```python
from build123d import *

# Parameters (mm, degrees)
F1_DEPTH  = 50
F2_R      = 20
F3_DEPTH  = 25
F6_R      = 0.75
F7_DEPTH  = 25
F9_DEPTH  = 2
F10_R     = 0.75
F11_DEPTH = 5


# Not quite as in the source:
# - the program builds the solid bodies; features that only make, move or delete a surface that nothing else refers to are left out


with BuildPart() as f1:
    # F0 (on Top) → F1 (new body)
    with BuildSketch(Plane.XY):
        with BuildLine():
            Line((16.436829567, 25), (-13.563170433, 25))
            ThreePointArc((-13.563170433, 25), (-20.6342382449, 22.0710678119), (-23.563170433, 15))
            Line((-23.563170433, 15), (-23.563170433, -15))
            ThreePointArc((-23.563170433, -15), (-20.6342382449, -22.0710678119), (-13.563170433, -25))
            Line((-13.563170433, -25), (16.436829567, -25))
            ThreePointArc((16.436829567, -25), (23.5078973788, -22.0710678119), (26.436829567, -15))
            Line((26.436829567, -15), (26.436829567, 15))
            ThreePointArc((26.436829567, 15), (23.5078973788, 22.0710678119), (16.436829567, 25))
        make_face()
    extrude(amount=F1_DEPTH)

    # F2 (on face) → F3 (cut)
    with BuildSketch(Plane.XY.offset(50)):
        Circle(F2_R)
    extrude(amount=-F3_DEPTH, mode=Mode.SUBTRACT)

    # F4 (on Front) → F5 (revolve, cut)
    with BuildSketch(Plane.XZ):
        Polygon((20, 48), (20, 50), (0, 50), (0, 25), (23, 25), (23, 48), align=None)
    revolve(axis=Axis((0, 0, 37.5), (0, 0, 1)), mode=Mode.SUBTRACT)

    # F6 (on face) → F7 (cut)
    with BuildSketch(Plane.XY.offset(50)):
        with Locations((0, 21.75)):
            Circle(F6_R)
        with Locations((0, -21.75)):
            Circle(F6_R)
    extrude(amount=-F7_DEPTH, mode=Mode.SUBTRACT)

    # F8 (on face) → F9 (cut)
    with BuildSketch(Plane.XY.offset(25)):
        with BuildLine():
            ThreePointArc((7, 4), (6.7071067812, 4.7071067812), (6, 5))
            Line((6, 5), (-6, 5))
            ThreePointArc((-6, 5), (-6.7071067812, 4.7071067812), (-7, 4))
            Line((-7, 4), (-7, -4))
            ThreePointArc((-7, -4), (-6.7071067812, -4.7071067812), (-6, -5))
            Line((-6, -5), (6, -5))
            ThreePointArc((6, -5), (6.7071067812, -4.7071067812), (7, -4))
            Line((7, -4), (7, 4))
        make_face()
    extrude(amount=-F9_DEPTH, mode=Mode.SUBTRACT)

    # F10 (on face) → F11 (cut)
    with BuildSketch(Plane.XY.offset(23)):
        with Locations((-5.4101994716, 3.5321465987)):
            Circle(F10_R)
        with Locations((-5.4101994716, -3.5321465987)):
            Circle(F10_R)
        with Locations((5.4101994716, 3.5321465987)):
            Circle(F10_R)
        with Locations((5.4101994716, -3.5321465987)):
            Circle(F10_R)
    extrude(amount=-F11_DEPTH, mode=Mode.SUBTRACT)


solid = f1.part
```
Here's how the part is built. I have some questions about the finished solid (model axes, mm). A direction names the side the tool comes from. Give positions to 0.01 mm unless a question says otherwise; leave off trailing zeros. Loops run counter-clockwise (first coordinate to the right, second up) from the corner with the lowest first, then second, coordinate; pieces in that order, holes last. Notation, with made-up numbers: M 8,-37.5 L 43,-37.5 A25 cw 43,-8.5 Z; hole C 28,-18.75 d10. An arc over 180 degrees is marked long. Use one line per item in the form item = value. Start each with the question number.
Q1. If we section it at B-B (x = 0): Write out the boundary of the cut face in (y, z), then the cut area to 3 significant figures.
Q2. If we section it at A-A (z = 33): Write out the boundary of the cut face in (x, y), then the cut area to 3 significant figures.
Q3. Will these pins go through, and if not, where does the flat tip stop? pin 1 Ø12 at (x, y) = (-7, -10.5) entering from +Z; pin 2 Ø1.2 at (x, y) = (5.41, 3.53) entering from -Z; pin 3 Ø1.2 at (x, y) = (-5.41, -3.53) entering from +Z; pin 4 Ø2 at (x, z) = (-17.5, 34.5) entering from +Y.
Q4. Thinking about a two-plate mould opening in Y: for faces 1 (the cylindrical face through (5.31, -2.79, 20.54)), 2 (the flat face through (7, 0, 24)), 3 (the flat face through (-23.563, 0, 25)), 4 (the cylindrical face through (-20.556, 22.148, 24.65)), which applies, +Y half, -Y half, draft (parallel to the pull), parting line (faces both ways), or undercut?
Q5. If we section it at D-D (y = 0): Write out the boundary of the cut face in (x, z).
Q6. I need wall thicknesses on line 1 along Z through (x, y) = (9, -19); line 2 along Z through (x, y) = (11.5, 8.5); line 3 along X through (y, z) = (-17, 27.5). Which ranges of each line are inside material? Lowest first, please.
Q7. If we section it at C-C (z = 8): Write out the boundary of the cut face in (x, y).
Q8. Which directions (+Z, -Z, +X, -X, +Y, -Y) give clear straight access to the entire face, cutting with the end or side of a thin tool? Please do faces 5 (the flat face through (26.437, 0, 25)), 6 (the cylindrical face through (-2.994, 22.804, 36.661)), 7 (the cylindrical face through (0, 21, 49)).
Taken from the geometry:
q1.outline = M -25,0 L 25,0 L 25,50 L 22.5,50 L 22.5,48 L 23,48 L 23,25 L 5,25 L 5,23 L -5,23 L -5,25 L -23,25 L -23,48 L -22.5,48 L -22.5,50 L -25,50 Z; M -21,48 L -20,48 L -20,50 L -21,50 Z; M 20,48 L 21,48 L 21,50 L 20,50 Z
q1.area = 1,340 mm^2
q2.outline = M -23.56,-15 A10 ccw -13.56,-25 L 16.44,-25 A10 ccw 26.44,-15 L 26.44,15 A10 ccw 16.44,25 L -13.56,25 A10 ccw -23.56,15 Z; hole C 0,0 d46
q2.area = 752 mm^2
q3.pin_1 = 25
q3.pin_2 = 0
q3.pin_3 = 18
q3.pin_4 = 24.56
q4.face_1 = undercut
q4.face_2 = undercut
q4.face_3 = draft
q4.face_4 = +Y half
q5.outline = M -23.56,0 L 26.44,0 L 26.44,50 L 20,50 L 20,48 L 23,48 L 23,25 L 7,25 L 7,23 L -7,23 L -7,25 L -23,25 L -23,48 L -20,48 L -20,50 L -23.56,50 Z
q6.line_1 = 0 to 25, 48 to 50
q6.line_2 = 0 to 25
q6.line_3 = -23.36 to -15.49, 15.49 to 26.23
q7.outline = M -23.56,-15 A10 ccw -13.56,-25 L 16.44,-25 A10 ccw 26.44,-15 L 26.44,15 A10 ccw 16.44,25 L -13.56,25 A10 ccw -23.56,15 Z
q8.face_5 = +Z, -Z, +X, +Y, -Y
q8.face_6 = none
q8.face_7 = +Z
